Could you check a few things on this model? Use its own coordinates, in mm. Coordinates: 2 decimals unless noted, no trailing zeros. Loops run counter-clockwise (first coordinate to the right, second up) from the corner with the lowest first, then second, coordinate; pieces in that order, holes last. Notation, with made-up numbers: M 49,65 L 71,65 A23 cw 71,78 Z; hole C 18,14 d10. An arc over 180 degrees is marked long. Return JSON: item names as keys, results as strings. Group by question number.
from build123d import *

# Parameters (mm, degrees)
F1_DEPTH = 25
F2_DEPTH = 5


with BuildPart() as f1:
    # F0 (on Front) → F1 (new body)
    with BuildSketch(Plane.XZ):
        with BuildLine():
            Line((25, -20), (25, 25))
            Line((25, 25), (-25, 25))
            Line((-25, 25), (-25, -25))
            Line((-25, -25), (20, -25))
            ThreePointArc((20, -25), (16.464466, -16.464466), (25, -20))
        make_face()
        with BuildLine():
            Line((25, -25), (25, -20))
            ThreePointArc((25, -20), (23.535534, -23.535534), (20, -25))
            Line((20, -25), (25, -25))
        make_face()
        with BuildLine():
            ThreePointArc((20, -25), (23.535534, -23.535534), (25, -20))
            ThreePointArc((25, -20), (16.464466, -16.464466), (20, -25))
        make_face()
    extrude(amount=F1_DEPTH)

    # F0 (on Front) → F2 (join)
    with BuildSketch(Plane.XZ):
        with BuildLine():
            ThreePointArc((20, -25), (23.535534, -23.535534), (25, -20))
            ThreePointArc((25, -20), (16.464466, -16.464466), (20, -25))
        make_face()
    extrude(amount=-F2_DEPTH)


solid = f1.part
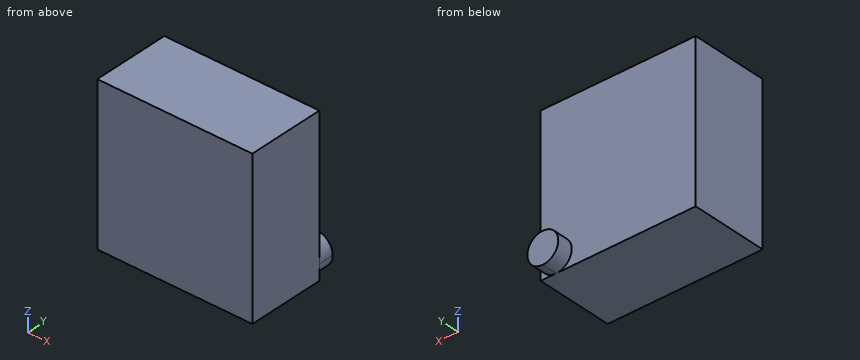
(1) Will this pin go through, and if not, where does the flat tip stop? P1, Ø12, axis at x = -17, z = -16.5, coming from the +Y side.
(2) Imagine slicing it at B-B, the plane z = 1.5. Write out the boundary of the cut face in (x, y).
(3) If I drill on L1, parallel to Y at x = -11, z = -2, over which ranges is the centre line in solid material (lowest first)? Write a range as [from, to].
(4) Imagine slicing it at C-C, the plane x = -5.5. Write out the boundary of the cut face in (y, z), then the cut area to 3 significant figures.
(5) Imagine slicing it at A-A, the plane x = 17. Write out the boundary of the cut face in (y, z), then the cut area to 3 significant figures.
Checks:
{
 "1": {"P1": "y = 0"},
 "2": {"outline": "M -25,-25 L 25,-25 L 25,0 L -25,0 Z"},
 "3": {"L1": "[-25, 0]"},
 "4": {"outline": "M -25,-25 L 0,-25 L 0,25 L -25,25 Z", "area": "1,250 mm²"},
 "5": {"outline": "M -25,-25 L 0,-25 L 0,-24 L 5,-24 L 5,-16 L 0,-16 L 0,25 L -25,25 Z", "area": "1,290 mm²"}
}
